Part model, mm, in its own coordinate system. Face numbers are marked on the shaded views. A direction names the side the tool comes from. Round coordinates to 2 decimals unless told otherwise and drop trailing zeros. Loops run counter-clockwise (first coordinate to the right, second up) from the corner with the lowest first, then second, coordinate; pieces in that order, holes last.
1) Probe line 1 (Z direction, x = 3.55, y = 23); line 2 (Y direction, x = 1.5, z = -9); line 3 (Z direction, x = 11, y = -25). List the from-to ranges inside material, lowest first.
2) Drop flat-ended pins along their axis: P1, Ø1, axis at x = 6, z = 46, coming from the +Y side; P2, Ø5, axis at x = 11, y = -22, coming from the +Z side; P3, Ø1.5, axis at y = -16.5, z = 5.5, coming from the -X side; P4, Ø5, axis at y = -17, z = 50, coming from the -X side. Give the stop position or say it passes through.
3) Band-saw the part on B-B, the plane z = 27. Write the cut outline in (x, y).
4) 3-axis set-ups, long thin cutter, end or side, ignore diameter. For the marked faces 4, 5 and 6: which of +Z, -Z, +X, -X, +Y, -Y reach the whole face in a straight line?
5) Mould opens along Z. For the marked faces 1, 2 and 3 say: +Z half, -Z half, draft (parallel to the pull), parting line (faces both ways), or undercut.
6) Band-saw the part on A-A, the plane y = 14. Write the cut outline in (x, z).
7) Band-saw the part on C-C, the plane x = 8.25. State how many separate pieces and enclosed holes the cut face has, then the cut area to 3 significant figures.
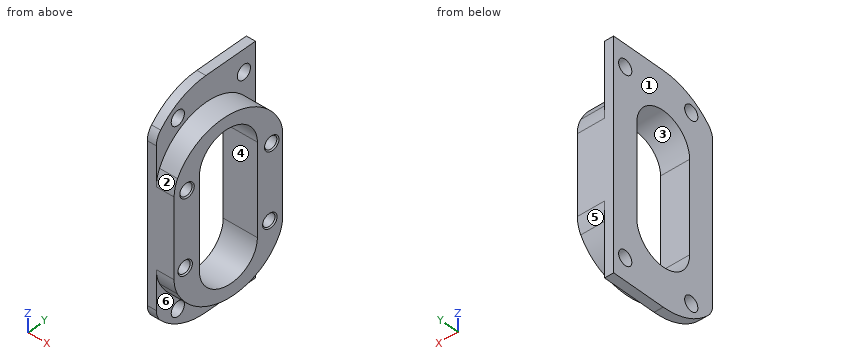
from build123d import *

# Parameters (mm, degrees)
SZKIC1_R                                   = 4
DODANIE_WYCI_GNI_CIE1_DEPTH                = 20
SZKIC2_OUTSIDE_W                           = 153.84
SZKIC2_OUTSIDE_H                           = 89.84
WYTNIJ_WYCI_GNI_CIE1_DEPTH                 = 15
WYTNIJ_WYCI_GNI_CIE2_DEPTH                 = 130.135587659
WYTNIJ_WYCI_GNI_CIE2_DEPTH_BACK            = 130.135587659
OTW_R_GWINTOWANY_M81_D                     = 6.8
OTW_R_GWINTOWANY_M81_DEPTH                 = 12.957073895
OTW_R_GWINTOWANY_M81_CSINK_D               = 8.05
OTW_R_GWINTOWANY_M81_CSINK_ANGLE           = 90
OTW_R_GWINTOWANY_M81_TIP                   = 2.042926105
OTW_R_GWINTOWANY_M81_ON_FACE_2_D           = 6.8
OTW_R_GWINTOWANY_M81_ON_FACE_2_DEPTH       = 12.957073895
OTW_R_GWINTOWANY_M81_ON_FACE_2_CSINK_D     = 8.05
OTW_R_GWINTOWANY_M81_ON_FACE_2_CSINK_ANGLE = 90
OTW_R_GWINTOWANY_M81_ON_FACE_2_TIP         = 2.042926105


with BuildPart() as part:
    # Szkic1 → Dodanie-wyciągnięcie1 (new body)
    with BuildSketch(Plane(origin=(0, 0, 0), x_dir=(0, 0, -1), z_dir=(1, 0, 0))):
        with BuildLine():
            Line((-43.138357147, -30), (43.138357147, -30))
            ThreePointArc((43.138357147, -30), (46.738768646, -29.329364235), (49.856267202, -27.407407407))
            ThreePointArc((49.856267202, -27.407407407), (58.828108774, -14.988630917), (62, 0))
            Line((62, 0), (62, 30))
            Line((62, 30), (-62, 30))
            Line((-62, 30), (-62, 0))
            ThreePointArc((-62, 0), (-58.828108774, -14.988630917), (-49.856267202, -27.407407407))
            ThreePointArc((-49.856267202, -27.407407407), (-46.738768646, -29.329364235), (-43.138357147, -30))
        make_face()
        with Locations((-50, 23)):
            Circle(SZKIC1_R, mode=Mode.SUBTRACT)
        with Locations((50, 23)):
            Circle(SZKIC1_R, mode=Mode.SUBTRACT)
        with Locations((50, -17)):
            Circle(SZKIC1_R, mode=Mode.SUBTRACT)
        with Locations((-50, -17)):
            Circle(SZKIC1_R, mode=Mode.SUBTRACT)
        with BuildLine():
            Line((-25, -16), (25, -16))
            ThreePointArc((25, -16), (41, 0), (25, 16))
            Line((25, 16), (-25, 16))
            ThreePointArc((-25, 16), (-41, 0), (-25, -16))
        make_face(mode=Mode.SUBTRACT)
    extrude(amount=DODANIE_WYCI_GNI_CIE1_DEPTH)

    # Szkic2 outside → Wytnij-wyciągnięcie1 (cut)
    # profile 1 of 2: a face of its own
    with BuildSketch(Plane(origin=(20, 0, 0), x_dir=(0, 0, -1), z_dir=(1, 0, 0))):
        Rectangle(SZKIC2_OUTSIDE_W, SZKIC2_OUTSIDE_H)
        with BuildLine():
            Line((21.671768561, 30), (-21.671768561, 30))
            ThreePointArc((-21.671768561, 30), (-26.059642547, 29.512728202), (-30.233707808, 28.074656189))
            ThreePointArc((-30.233707808, 28.074656189), (-48, 0), (-30.233707808, -28.074656189))
            ThreePointArc((-30.233707808, -28.074656189), (-26.059642547, -29.512728202), (-21.671768561, -30))
            Line((-21.671768561, -30), (21.671768561, -30))
            ThreePointArc((21.671768561, -30), (26.059642547, -29.512728202), (30.233707808, -28.074656189))
            ThreePointArc((30.233707808, -28.074656189), (48, 0), (30.233707808, 28.074656189))
            ThreePointArc((30.233707808, 28.074656189), (26.059642547, 29.512728202), (21.671768561, 30))
        make_face(mode=Mode.SUBTRACT)
    # profile 2 of 2: a face of its own
    with BuildSketch(Plane(origin=(20, 0, 0), x_dir=(0, 0, -1), z_dir=(1, 0, 0))):
        with BuildLine():
            Line((-25, -16), (25, -16))
            ThreePointArc((25, -16), (41, 0), (25, 16))
            Line((25, 16), (-25, 16))
            ThreePointArc((-25, 16), (-41, 0), (-25, -16))
        make_face()
    extrude(amount=-WYTNIJ_WYCI_GNI_CIE1_DEPTH, mode=Mode.SUBTRACT)

    # Szkic3 → Wytnij-wyciągnięcie2 (cut, two sides: drawn at the far end of the back side and taken through both)
    with BuildSketch(Plane(origin=(0, 0, -62), x_dir=(-1, 0, 0), z_dir=(0, 0, -1)).offset(-WYTNIJ_WYCI_GNI_CIE2_DEPTH_BACK)):
        Polygon((-20, 30), (-14.750680188, -30), (-20, -30), align=None)
    extrude(amount=WYTNIJ_WYCI_GNI_CIE2_DEPTH + WYTNIJ_WYCI_GNI_CIE2_DEPTH_BACK, mode=Mode.SUBTRACT)

    # Otwór gwintowany M81
    with Locations(Plane(origin=(19.469847212, 23.940325899, 20), x_dir=(0.087155742748, 0.996194698092, 0), z_dir=(0.996194698092, -0.087155742748, 0))):
        with Locations((0, 0), (-1.047077932, -39.986292999)):
            CounterSinkHole(OTW_R_GWINTOWANY_M81_D / 2, OTW_R_GWINTOWANY_M81_CSINK_D / 2, depth=OTW_R_GWINTOWANY_M81_DEPTH, counter_sink_angle=OTW_R_GWINTOWANY_M81_CSINK_ANGLE)
            with Locations((0, 0, -(OTW_R_GWINTOWANY_M81_DEPTH + OTW_R_GWINTOWANY_M81_TIP / 2))):  # 118° drill point
                Cone(0, OTW_R_GWINTOWANY_M81_D / 2, OTW_R_GWINTOWANY_M81_TIP, mode=Mode.SUBTRACT)

    # Otwór gwintowany M81 on face 2
    with Locations(Plane(origin=(15.374931009, -22.864780472, 21.23031657), x_dir=(0.087155971833, 0.996194678049, 0), z_dir=(0.996194678049, -0.087155971833, 0))):
        with Locations((0, 0), (-1.047077932, -39.986292999)):
            CounterSinkHole(OTW_R_GWINTOWANY_M81_ON_FACE_2_D / 2, OTW_R_GWINTOWANY_M81_ON_FACE_2_CSINK_D / 2, depth=OTW_R_GWINTOWANY_M81_ON_FACE_2_DEPTH, counter_sink_angle=OTW_R_GWINTOWANY_M81_ON_FACE_2_CSINK_ANGLE)
            with Locations((0, 0, -(OTW_R_GWINTOWANY_M81_ON_FACE_2_DEPTH + OTW_R_GWINTOWANY_M81_ON_FACE_2_TIP / 2))):  # 118° drill point
                Cone(0, OTW_R_GWINTOWANY_M81_ON_FACE_2_D / 2, OTW_R_GWINTOWANY_M81_ON_FACE_2_TIP, mode=Mode.SUBTRACT)


solid = part.part
Reported:
1. line 1: z = -62 to -54, -46 to 46, 54 to 62
1. line 2: y = -30 to -16, 16 to 30
1. line 3: z = -35.38 to -21.83, -15.69 to 18.94, 23.53 to 35.38
2. P1: stops at y = 12.21
2. P2: stops at z = 41.12
2. P3: stops at x = 0
2. P4: passes through
3. outline: (0, -30) - (5, -30) - (5, -29.28) - (14.81, -29.28) - (15.99, -15.87) - (0, -15.87) - close; (0, 15.87) - (18.76, 15.87) - (19.94, 29.28) - (5, 29.28) - (5, 30) - (0, 30) - close
4. face 4: +X, -X
4. face 5: -Z, +X, +Y
4. face 6: -Z, +X
5. face 1: draft
5. face 2: +Z half
5. face 3: undercut
6. outline: (0, -62) - (5, -62) - (5, -44.67) - (18.6, -44.67) - (18.6, -32.75) - (0, -32.75) - close; (0, 32.75) - (18.6, 32.75) - (18.6, 44.67) - (5, 44.67) - (5, 62) - (0, 62) - close
7. separate pieces: 1
7. enclosed holes: 5
7. area: 2,490 mm2
